Work out the finished part from the listing and answer in its coordinate system (mm). Face numbers are marked on the shaded views. A direction names the side the tool comes from. Round coordinates to 2 decimals unless told otherwise and drop trailing zeros. Write each loop counter-clockwise with the first axis right and the second up, starting at its lowest first coordinate (ties: lowest second). Pieces come first, ordered by that corner, then holes. Notation, with made-up numbers: (26, 89.5) -> (52, 89.5) arc R20 ccw to (52, 108.5) -> close; hole circle Ø4 at (-30, 80.25). An arc over 180 degrees is marked (long way). Answer as a JSON object with one key per item and string values. Group by question number.
from build123d import *

# Parameters (mm, degrees)
F1_DEPTH = 35
F2_R     = 12
F3_R     = 5
F4_DEPTH = 25.4
F6_D     = 10


with BuildPart() as f1:
    # F0 (on Front) → F1 (new body, symmetric)
    with BuildSketch(Plane.XZ):
        Polygon((38, 0), (0, 0), (0, -12), (44, -12), (44, -8), (92, -8), (92, -12), (136, -12), (136, 0), (98, 0), (98, 4), (68, 4), (38, 4), align=None)
    extrude(amount=F1_DEPTH, both=True)

    # F2
    f2_edges = [f1.edges().sort_by_distance(p)[0] for p in [
        (0, -35, -6),
        (136, -35, -6),
        (136, 35, -6),
        (0, 35, -6),
    ]]
    fillet(f2_edges, radius=F2_R)

    # F3 (on face) → F4 (cut)
    with BuildSketch(Plane.XY):
        with Locations((12, 23)):
            Circle(F3_R)
        with Locations((12, -23)):
            Circle(F3_R)
    extrude(amount=-F4_DEPTH, mode=Mode.SUBTRACT)

    # F6 (through all)
    with Locations(Plane.XY):
        with Locations((124, 23), (124, -23)):
            Hole(F6_D / 2)


solid = f1.part
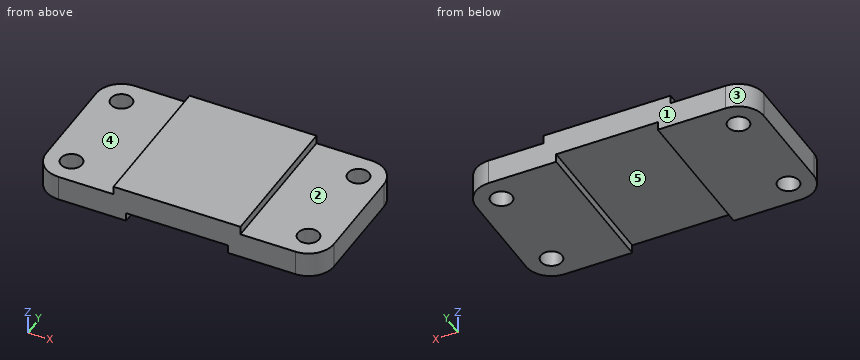
1) Straight lines are drawn through the part: L1, parallel to Y at x = 124, z = -2.5; L2, parallel to X at y = 17, z = -10; L3, parallel to X at y = 21, z = -0.25. For each, find the intervals that lie inside material, in ascending order.
2) A cutting plane is placed at D-D on x = 54. Determine the outline of the cut face in (y, z), plus the area to 3 significant figures.
3) A tool of negligible diameter and unlimited length cuts with its end or side. For the marked faces 1 and 2, from which of +Z, -Z, +X, -X, +Y, -Y can it reach the whole face along a straight path? Write none if from no direction.
4) A cutting plane is placed at A-A on z = -10.25. Determine the outline of the cut face in (x, y).
5) For a pull along X with two mould halves and no side action, classify the marked faces 3, 4 and 5 as released by +X, released by -X, zero draft, split by the parting line, or undercut.
6) A cutting plane is placed at C-C on z = -4.75. Determine the outline of the cut face in (x, y), plus the area to 3 significant figures.
7) A cutting plane is placed at B-B on y = -12. Determine the outline of the cut face in (x, z), plus the area to 3 significant figures.
8) Each of these flat-tipped pins is pushed along its axis until it touches: P1, Ø16, axis at x = 12, y = -23, coming from the +Z side; P2, Ø14.5, axis at x = 63.5, y = 6.5, coming from the -Z side; P3, Ø3, axis at y = 13.5, z = 2, coming from the -X side. Where does it stop, or does it pass through?
Established:
{
 "1": {"L1": "y = -35 to -28, -18 to 18, 28 to 35", "L2": "x = 0 to 44, 92 to 136", "L3": "x = 0 to 7.42, 16.58 to 119.42, 128.58 to 136"},
 "2": {"outline": "(-35, -8) -> (35, -8) -> (35, 4) -> (-35, 4) -> close", "area": "840 mm²"},
 "3": {"face 1": "+Z, -Z, +X, -X, +Y", "face 2": "+Z, +X, +Y, -Y"},
 "4": {"outline": "(0, -23) arc R12 ccw to (12, -35) -> (44, -35) -> (44, 35) -> (12, 35) arc R12 ccw to (0, 23) -> close; (92, -35) -> (124, -35) arc R12 ccw to (136, -23) -> (136, 23) arc R12 ccw to (124, 35) -> (92, 35) -> close; hole circle Ø10 at (12, -23); hole circle Ø10 at (12, 23); hole circle Ø10 at (124, -23); hole circle Ø10 at (124, 23)"},
 "5": {"face 3": "released by -X", "face 4": "zero draft", "face 5": "undercut"},
 "6": {"outline": "(0, -23) arc R12 ccw to (12, -35) -> (124, -35) arc R12 ccw to (136, -23) -> (136, 23) arc R12 ccw to (124, 35) -> (12, 35) arc R12 ccw to (0, 23) -> close; hole circle Ø10 at (12, -23); hole circle Ø10 at (12, 23); hole circle Ø10 at (124, -23); hole circle Ø10 at (124, 23)", "area": "9,080 mm²"},
 "7": {"outline": "(0, -12) -> (44, -12) -> (44, -8) -> (92, -8) -> (92, -12) -> (136, -12) -> (136, 0) -> (98, 0) -> (98, 4) -> (38, 4) -> (38, 0) -> (0, 0) -> close", "area": "1,680 mm²"},
 "8": {"P1": "stops at z = 0", "P2": "stops at z = -8", "P3": "stops at x = 38"}
}
